Geometry check sheet. Reference: the model listing, model coordinates, mm. Face numbers are marked on the shaded views. A direction names the side the tool comes from. Round coordinates to 2 decimals unless told otherwise and drop trailing zeros. Write each loop counter-clockwise with the first axis right and the second up, starting at its lowest first coordinate (ties: lowest second). Pieces come first, ordered by that corner, then holes. Notation, with made-up numbers: M -15.5,82.5 L 30.5,82.5 A8 cw 30.5,95.5 Z; hole C -39,86.25 d5. An arc over 180 degrees is marked long. Put each result on its own line as item: value. Start each with the question number.
(1) Section check D-D on y = 35.5. Record the cut outline in (x, z).
(2) Section check C-C on z = 12. Record the cut outline in (x, y).
(3) Gauge pin test, flat ends, axial feed: pin 1 (11 mm diameter, centred on x = 20, z = 17.5, fed in from +Y); pin 2 (1.6 mm diameter, centred on x = 1, z = 6, fed in from +Y). Record the tip position at first contact, or that the pin passes through.
(4) Section check B-B on z = 30. Record the cut outline in (x, y).
(5) Section check A-A on x = 19. Record the cut outline in (y, z), then the cut area to 3 significant figures.
(6) Tool access check on the marked faces 1 and 2. Record the directions out of +Z, -Z, +X, -X, +Y, -Y that give a thin tool (end or side, any length) a straight path to the whole face; none if there is none.
(7) Material ranges on probe 1 along Y at (x, z) = (31, 22); probe 2 along Z at (x, y) = (19, 1.2), recorded low to high.
from build123d import *

# Parameters (mm, degrees)
EXTRUDE_1_DEPTH     = 60
SKETCH_2_R          = 1.5
SKETCH_2_R_2        = 3.5
CUT_EXTRUDE_1_DEPTH = 39
SKETCH_3_R          = 4
CUT_EXTRUDE_2_DEPTH = 50


with BuildPart() as part:
    # 草图1 → 凸台-拉伸1 (new body)
    with BuildSketch(Plane.XY):
        Polygon((0, 58), (0, 0), (38, 0), (38, 2), (2, 2), (2, 58), align=None)
    extrude(amount=EXTRUDE_1_DEPTH)

    # 草图2 → 切除-拉伸1 (cut, through all)
    with BuildSketch(Plane.ZY):
        with Locations((30.710851292, 54.912666943)):
            Circle(SKETCH_2_R)
        with Locations((40.948406341, 54.912666943)):
            Circle(SKETCH_2_R)
        with Locations((12, 33)):
            Circle(SKETCH_2_R_2)
        Polygon((60, 0), (60, 58), (48, 58), align=None)
        Polygon((26, 58), (21.884599262, 48), (0, 48), (0, 58), align=None)
    extrude(amount=-CUT_EXTRUDE_1_DEPTH, mode=Mode.SUBTRACT)

    # 草图3 → 切除-拉伸2 (cut)
    with BuildSketch(Plane.XZ):
        with Locations((19, 13.5)):
            Circle(SKETCH_3_R)
    extrude(amount=-CUT_EXTRUDE_2_DEPTH, mode=Mode.SUBTRACT)


solid = part.part
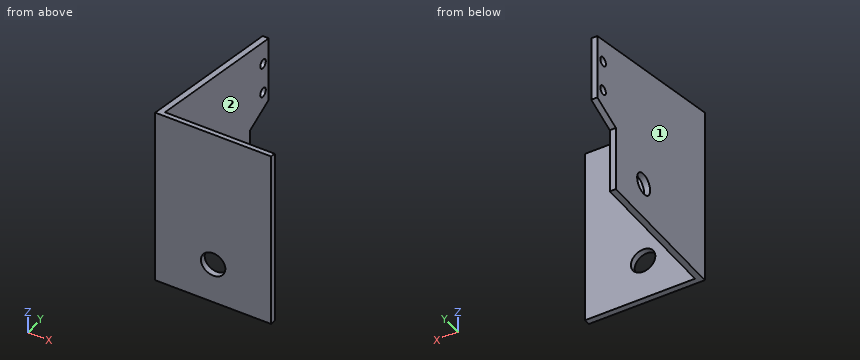
Answers follow:
1. outline: M 0,0 L 2,0 L 2,9.55 L 0,9.55 Z; M 0,14.45 L 2,14.45 L 2,52.66 L 0,52.66 Z
2. outline: M 0,0 L 15.29,0 L 15.29,2 L 2,2 L 2,29.5 L 0,29.5 Z; M 0,36.5 L 2,36.5 L 2,48 L 0,48 Z; M 22.71,0 L 38,0 L 38,2 L 22.71,2 Z
3. pin 1: stops at y = 2
3. pin 2: stops at y = 48
4. outline: M 0,0 L 38,0 L 38,2 L 2,2 L 2,53.59 L 0,53.59 Z; M 0,56.23 L 2,56.23 L 2,58 L 0,58 Z
5. outline: M 0,0 L 2,0 L 2,9.5 L 0,9.5 Z; M 0,17.5 L 2,17.5 L 2,59.59 L 0,60 Z
5. area: 104 mm^2
6. face 1: +Z, -Z, -X, +Y, -Y
6. face 2: +Z, -Z, +X, +Y
7. probe 1: y = 0 to 2
7. probe 2: z = 0 to 9.5, 17.5 to 59.75
